Input: part model. Units: mm. Frame: model coordinates. A direction names the side the tool comes from. Coordinates: 2 decimals unless noted, no trailing zeros. Loops run counter-clockwise (first coordinate to the right, second up) from the corner with the lowest first, then second, coordinate; pieces in that order, holes last.
(1) Section B-B, the plane y = 1.15. Return loops of the section in (x, z), then the cut area to 3 significant figures.
(2) Contact query for a flat-ended pin moving along its axis: P1, Ø0.6, axis at x = 0, y = 2, coming from the +Z side. Output: stop coordinate, or through.
(3) Section C-C, the plane x = 0. Return loops of the section in (y, z), then the cut area to 3 significant figures.
(4) Section A-A, the plane z = 13.5. Return loops of the section in (x, y), then the cut area to 3 significant figures.
(5) Mould query, pull axis X, two halves, no side actions, for faces 3 (the face through (-3.81, 2, 15)), 4 (the face through (16.1, 1.5, 16.3)), 5 (the face through (-16.1, 1.5, 16.3)), 6 (the face through (0, 2, -16.7)). Classes: released by +X, released by -X, zero draft, split by the parting line, or undercut.
(6) Line query: L1, parallel to X at y = 2.1, z = 13; L2, parallel to Z at x = 2, y = 2.15; L3, parallel to Z at x = 4, y = 0.15. Output: solid intervals per line, ascending.
(7) Set-up query: faces 1 (the face through (9, 2, 16.7)), 2 (the face through (3.81, 2, 15)). Return all of +Z, -Z, +X, -X, +Y, -Y with unobstructed straight access to the full face (end or side cutting, diameter ignored); none if empty.
```python
from build123d import *

# Parameters (mm, degrees)
BOSS_EXTRUDE1_DEPTH = 2.54
FILLET1_R           = 0.508


with BuildPart() as part:
    # Sketch1 → Boss-Extrude1 (new body)
    with BuildSketch(Plane(origin=(0, 0, 0), x_dir=(1, 0, 0), z_dir=(0, 1, 0))):
        with BuildLine():
            Line((-3.81, -16.7005), (-3.81, -12.8905))
            Line((-3.81, -12.8905), (3.81, -12.8905))
            Line((3.81, -12.8905), (3.81, -16.7005))
            Line((3.81, -16.7005), (15.1765, -16.7005))
            ThreePointArc((15.1765, -16.7005), (16.074525612, -16.328525612), (16.4465, -15.4305))
            Line((16.4465, -15.4305), (16.4465, 15.4305))
            ThreePointArc((16.4465, 15.4305), (16.074525612, 16.328525612), (15.1765, 16.7005))
            Line((15.1765, 16.7005), (-15.1765, 16.7005))
            ThreePointArc((-15.1765, 16.7005), (-16.074525612, 16.328525612), (-16.4465, 15.4305))
            Line((-16.4465, 15.4305), (-16.4465, -15.4305))
            ThreePointArc((-16.4465, -15.4305), (-16.074525612, -16.328525612), (-15.1765, -16.7005))
            Line((-15.1765, -16.7005), (-3.81, -16.7005))
        make_face()
    extrude(amount=BOSS_EXTRUDE1_DEPTH)

    # Fillet1
    fillet1_edges = [part.edges().sort_by_distance(p)[0] for p in [
        (-16.4465, 0, 0),
        (-16.074525612, 0, -16.328525612),
        (0, 0, -16.7005),
        (16.074525612, 0, -16.328525612),
        (16.4465, 0, 0),
        (16.074525612, 0, 16.328525612),
        (9.49325, 0, 16.7005),
        (3.81, 0, 14.7955),
        (0, 0, 12.8905),
        (-3.81, 0, 14.7955),
        (-9.49325, 0, 16.7005),
        (-16.074525612, 0, 16.328525612),
    ]]
    fillet(fillet1_edges, radius=FILLET1_R)


solid = part.part
```
Report:
1. outline: (-16.45, -15.43) arc R1.27 ccw to (-15.18, -16.7) - (15.18, -16.7) arc R1.27 ccw to (16.45, -15.43) - (16.45, 15.43) arc R1.27 ccw to (15.18, 16.7) - (3.81, 16.7) - (3.81, 12.89) - (-3.81, 12.89) - (-3.81, 16.7) - (-15.18, 16.7) arc R1.27 ccw to (-16.45, 15.43) - close
1. area: 1,070 mm2
2. P1: stops at z = 12.89
3. outline: (0, -16.19) arc R0.51 ccw to (0.51, -16.7) - (2.54, -16.7) - (2.54, 12.89) - (0.51, 12.89) arc R0.51 ccw to (0, 12.38) - close
3. area: 75.1 mm2
4. outline: (-16.45, 0.51) arc R0.51 ccw to (-15.94, 0) - (-4.32, 0) arc R0.51 ccw to (-3.81, 0.51) - (-3.81, 2.54) - (-16.45, 2.54) - close; (3.81, 0.51) arc R0.51 ccw to (4.32, 0) - (15.94, 0) arc R0.51 ccw to (16.45, 0.51) - (16.45, 2.54) - (3.81, 2.54) - close
4. area: 64.0 mm2
5. face 3: undercut
5. face 4: released by +X
5. face 5: released by -X
5. face 6: zero draft
6. L1: x = -16.45 to -3.81, 3.81 to 16.45
6. L2: z = -16.7 to 12.89
6. L3: z = -16.55 to 16.55
7. face 1: +Z, +X, -X, +Y, -Y
7. face 2: +Z, +Y, -Y
